Autodesk Inventor part; units mm, degrees
ref_plane "Work Plane1" through (0, 0, 33.3375) normal (0, 0, 1) x (1, 0, 0)
ref_plane "YZ Plane" through (0, 0, 0) normal (1, 0, 0) x (0, 1, 0)
ref_plane "XZ Plane" through (0, 0, 0) normal (0, 1, 0) x (-1, 0, 0)
sketch "Sketch1" plane through (0, 0, 0) normal (0, 0, 1) x (1, 0, 0)
  circle A0 centre (0, 0) radius 6.35
  dimension "d0" = 12.7
extrude "Extrusion1" add sketch "Sketch1" along normal blind 7.9375
sketch "Sketch2" plane through (0, 0, 7.9375) normal (0, 0, 1) x (1, 0, 0)
  circle A0 centre (0, 0) radius 6.35
  line L0 (-7.3323, 0) -> (-3.6662, 6.35)
  line L1 (-3.6662, 6.35) -> (3.6662, 6.35)
  line L2 (3.6662, 6.35) -> (7.3323, 0)
  line L3 (7.3323, 0) -> (3.6662, -6.35)
  line L4 (3.6662, -6.35) -> (-3.6662, -6.35)
  line L5 (-3.6662, -6.35) -> (-7.3323, 0)
  dimension "d4" = 12.7
extrude "Extrusion2" add sketch "Sketch2" along normal blind 50.8
sketch "Sketch3" plane through (0, 0, 58.7375) normal (0, 0, 1) x (1, 0, 0)
  circle A0 centre (0, 0) radius 6.35
  dimension "d7" = 12.7
extrude "Extrusion3" add sketch "Sketch3" along normal blind 7.9375
ref_plane "Work Plane1" through (0, 0, 33.3375) normal (0, 0, 1) x (1, 0, 0)
sketch "Sketch4" plane through (0, 0, 66.675) normal (0, 0, 1) x (1, 0, 0)
  circle A0 centre (0, 0) radius 6.35
  circle A1 centre (0, 0) radius 5.9436
  dimension "d10" = 11.8872
extrude "Extrusion4" add sketch "Sketch4" along normal blind 0.9906 contours A1
sketch "Sketch5" plane through (0, 0, 67.6656) normal (0, 0, 1) x (1, 0, 0)
  circle A0 centre (0, 0) radius 5.9436
  circle A1 centre (0, 0) radius 6.35
  dimension "d14" = 12.7
extrude "Extrusion5" add sketch "Sketch5" along normal blind 1.27 contours A0 | A1
mirror "Mirror1" about plane through (0, 0, 33.3375) normal (0, 0, 1) of "Extrusion4", "Extrusion5"
properties part number "Carriage Shaft - Lower" material "Aluminum 6061"
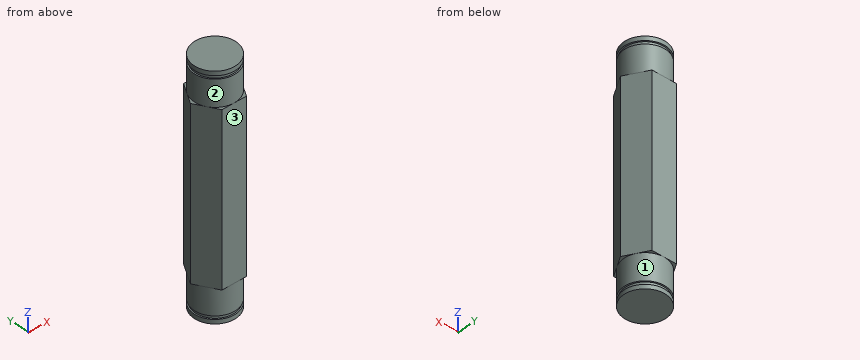
The model under review builds one solid part; all positions refer to its coordinate system, in mm. Face numbers are marked on the shaded views. A direction names the side the tool comes from. Round coordinates to 2 decimals unless told otherwise and drop trailing zeros. Loops run counter-clockwise (first coordinate to the right, second up) from the corner with the lowest first, then second, coordinate; pieces in that order, holes last. Notation, with made-up numbers: (18, 34.25) - (34, 34.25) arc R30 cw to (34, 62.25) - close; hole circle Ø7 at (81.25, 76.5). An arc over 180 degrees is marked (long way). Write each question's results on one line, items separated by ' | '. Start each with the question number.
Q1. Tool access review of the marked faces 1, 2 and 3: name each direction out of +Z, -Z, +X, -X, +Y, -Y from which nothing blocks a thin tool from reaching the whole face with its end or side.
Q2. Wall thickness on line 1 along Z through (x, y) = (-5, -3.5) (3 decimals); line 2 along Z through (x, y) = (6, 2.25); line 3 along X through (y, z) = (0, 4.5): over which ranges is each line inside the solid? List them lowest first. Write a range as [from, to].
Q3. Take a section at D-D on z = 62. Give the boundary of the cut face in (x, y).
Q4. Insertion check: P1, Ø0.9, axis at x = -6.5, y = 0.5, coming from the -Z side; P2, Ø1, axis at y = -5, z = 55, coming from the -X side; P3, Ø4, axis at y = 4.5, z = 39.5, coming from the +X side. Each pin has a flat end and moves straight along its axis. Give the tip position at first contact, or say it passes through.
Q5. Take a section at A-A on z = 11. Give the boundary of the cut face in (x, y).
Data:
1) face 1: -Z | face 2: +Z | face 3: +Z, -Z, +X, -X, -Y
2) line 1: z = [-2.261, -0.991], [0, 66.675], [67.666, 68.936] | line 2: z = [7.94, 58.74] | line 3: x = [-6.35, 6.35]
3) outline: circle Ø12.7 at (0, 0)
4) P1: stops at z = -2.26 | P2: stops at x = -4.73 | P3: stops at x = 5.89
5) outline: (-7.33, 0) - (-3.67, -6.35) - (3.67, -6.35) - (7.33, 0) - (3.67, 6.35) - (-3.67, 6.35) - close
